Geometry: final body of the model. Coordinates: model frame, mm. A direction names the side the tool comes from. Coordinates: 2 decimals unless noted, no trailing zeros. Order: outer loops, then holes, each group sorted by start corner. A loop starts at its lowest first (then second) coordinate and runs counter-clockwise, first axis right, second up. Notation, with made-up numbers: (44.5, 59) - (94.5, 59) arc R27 cw to (94.5, 98) - close; hole circle Ø10 at (52, 87.5). An arc over 180 degrees is marked (long way). Use a Markdown table: item, result. Add a question column.
```python
from build123d import *
from build123d.topology import SkipClean

# Parameters (mm, degrees)
EXTRUDE_1_DEPTH        = 15
SKETCH_4_W             = 25
SKETCH_4_H             = 29
CUT_EXTRUDE_2_DEPTH    = 13
PATTERN_LINEAR_1_COUNT = 4
PATTERN_LINEAR_1_PITCH = 27
CUT_EXTRUDE_3_DEPTH    = 149.559752288
EXTRUDE_2_DEPTH        = 142
CUT_EXTRUDE_4_DEPTH    = 149.559752288
SKETCH_14_W            = 21
SKETCH_14_H            = 4
CUT_EXTRUDE_7_DEPTH    = 84.348665256
PATTERN_LINEAR_3_COUNT = 5
PATTERN_LINEAR_3_PITCH = 27
CUT_EXTRUDE_8_DEPTH    = 84.348665256
SKETCH_17_R            = 2.5
CUT_EXTRUDE_9_DEPTH    = 84.348665256
PATTERN_LINEAR_4_COUNT = 4
PATTERN_LINEAR_4_PITCH = 27
SKETCH_21_W            = 31
SKETCH_21_H            = 13
CUT_EXTRUDE_11_DEPTH   = 32
CUT_EXTRUDE_12_DEPTH   = 0.5
PATTERN_LINEAR_5_COUNT = 4
PATTERN_LINEAR_5_PITCH = 27
CUT_EXTRUDE_13_DEPTH   = 6


# Read off the part's stored shape, not the designer's step: 镜向1
with BuildPart() as part:
    # 草图3 → 凸台-拉伸1 (new body)
    with BuildSketch(Plane(origin=(0, 0, 0), x_dir=(1, 0, 0), z_dir=(0, 1, 0))):
        Polygon((0, 0), (-71, 0), (-71, 41), (71, 41), (71, 0), align=None)
    extrude(amount=EXTRUDE_1_DEPTH)

    # 草图4 → 切除-拉伸2 (cut)
    with BuildSketch(Plane(origin=(0, 0, 0), x_dir=(1, 0, 0), z_dir=(0, 1, 0))):
        with Locations((-56.5, 24.5)):
            Rectangle(SKETCH_4_W, SKETCH_4_H)
    cut_extrude_2 = extrude(amount=CUT_EXTRUDE_2_DEPTH, mode=Mode.SUBTRACT)

    # 阵列(线性)1: 切除-拉伸2 ×4
    with Locations(*[(i * PATTERN_LINEAR_1_PITCH, 0, 0) for i in range(1, PATTERN_LINEAR_1_COUNT)]):
        add(cut_extrude_2, mode=Mode.SUBTRACT)

    # 草图6 → 切除-拉伸3 (cut, through all)
    with BuildSketch(Plane(origin=(71, 0, 0), x_dir=(0, 0, -1), z_dir=(1, 0, 0))):
        Polygon((0, 15), (7.5, 15), (8, 15), (8, 2), (7.5, 2), (0, 2), align=None)
    extrude(amount=-CUT_EXTRUDE_3_DEPTH, mode=Mode.SUBTRACT)

    # 草图7 → 凸台-拉伸2 (add)
    with BuildSketch(Plane(origin=(71, 0, 0), x_dir=(0, 0, -1), z_dir=(1, 0, 0))):
        with BuildLine():
            Line((0, 0), (4, 0))
            ThreePointArc((4, 0), (2.828427125, -2.828427125), (0, -4))
            Line((0, -4), (0, 0))
        make_face()
    extrude(amount=-EXTRUDE_2_DEPTH)

    # 草图8 → 切除-拉伸4 (cut, through all)
    with BuildSketch(Plane(origin=(71, 0, 0), x_dir=(0, 0, -1), z_dir=(1, 0, 0))):
        with BuildLine():
            Line((0, -1), (0, -2))
            Line((0, -2), (0, -3))
            ThreePointArc((0, -3), (1, -2), (0, -1))
        make_face()
    extrude(amount=-CUT_EXTRUDE_4_DEPTH, mode=Mode.SUBTRACT)

    # 草图14 → 切除-拉伸7 (cut, through all)
    with BuildSketch(Plane.XY):
        with Locations((-56.5, -2)):
            Rectangle(SKETCH_14_W, SKETCH_14_H)
    cut_extrude_7 = extrude(amount=-CUT_EXTRUDE_7_DEPTH, mode=Mode.SUBTRACT)

    # 阵列(线性)3: 切除-拉伸7 ×5
    with Locations(*[(i * PATTERN_LINEAR_3_PITCH, 0, 0) for i in range(1, PATTERN_LINEAR_3_COUNT)]):
        add(cut_extrude_7, mode=Mode.SUBTRACT)

    # 草图16 → 切除-拉伸8 (cut, through all)
    with BuildSketch(Plane.XY):
        Polygon((71, -1), (71, 0), (42.178247133, 0), (42.178247133, -4), (71, -4), align=None)
    extrude(amount=-CUT_EXTRUDE_8_DEPTH, mode=Mode.SUBTRACT)

    # 草图17 → 切除-拉伸9 (cut, through all)
    with BuildSketch(Plane.XZ):
        with Locations(Location((-56.5, -4, 0), (0, 0, 270))):
            Circle(SKETCH_17_R)
    cut_extrude_9 = extrude(amount=-CUT_EXTRUDE_9_DEPTH, mode=Mode.SUBTRACT)

    # 阵列(线性)4: 切除-拉伸9 ×4
    with Locations(*[(i * PATTERN_LINEAR_4_PITCH, 0, 0) for i in range(1, PATTERN_LINEAR_4_COUNT)]):
        add(cut_extrude_9, mode=Mode.SUBTRACT)

    # 草图21 → 切除-拉伸11 (cut)
    with BuildSketch(Plane(origin=(71, 0, 0), x_dir=(0, 0, -1), z_dir=(1, 0, 0))):
        with Locations((23.5, 8.5)):
            Rectangle(SKETCH_21_W, SKETCH_21_H)
    extrude(amount=-CUT_EXTRUDE_11_DEPTH, mode=Mode.SUBTRACT)

    # 草图23 → 切除-拉伸12 (cut)
    with BuildSketch(Plane(origin=(0, 0, -41), x_dir=(-1, 0, 0), z_dir=(0, 0, -1))):
        Polygon((55.25, 2.9), (56.5, 2.9), (57.75, 2.9), (57.75, 3.5), (57.75, 4.1), (55.25, 4.1), (55.25, 3.5), align=None)
    cut_extrude_12 = extrude(amount=-CUT_EXTRUDE_12_DEPTH, mode=Mode.SUBTRACT)

    # 阵列(线性)5: 切除-拉伸12 ×4
    with Locations(*[(i * PATTERN_LINEAR_5_PITCH, 0, 0) for i in range(1, PATTERN_LINEAR_5_COUNT)]):
        add(cut_extrude_12, mode=Mode.SUBTRACT)

    # 镜向1: part across plane


with BuildPart() as part_1:
    with SkipClean():  # the faces are left unmerged after this step: merging them gives an invalid solid
        add(part.part)
        add(part.part.mirror(Plane.XY))

    # 草图25 → 切除-拉伸13 (cut)
    with SkipClean():  # the faces are left unmerged after this step: merging them gives an invalid solid
        with BuildSketch(Plane(origin=(71, 0, 0), x_dir=(0, 0, -1), z_dir=(1, 0, 0))):
            Polygon((41, 15), (41, 0), (-41, 0), (-41, 15), (-39, 15), (-39, 2), (39, 2), (39, 15), align=None)
        extrude(amount=-CUT_EXTRUDE_13_DEPTH, mode=Mode.SUBTRACT)


solid = part_1.part
```
1) Draft query along Z for faces 6 (the flat face through (35, -0.7, -0.1)), 7 (the flat face through (24, 6, 10)), 8 (the flat face through (-3, 6, -39)). Return one class per face: released by +Z, released by -Z, zero draft, split by the parting line, or undercut.
2) Section query A-A (y = 8.5). Give the number of separate pieces and of enclosed holes in the cut face, and give its area (3 significant figures).
3) Section query B-B (z = 21.5). Return the cut outline in (x, y), and give its area (3 significant figures).
4) Access query for faces 1 (the flat face through (39, 9, 23)), 2 (the cylindrical face through (-4.94, 0.99, -3.46)), 3 (the flat face through (-13, -0.7, -0.1)), 4 (the flat face through (-3, 13, -25)), 5 (the flat face through (-15, 9, -8)). Directions: +Z, -Z, +X, -X, +Y, -Y. A direction counts if a zero-diameter tool reaches every point of the face in a straight line with its end or side. Return the directions, or none.
5) Line query: line 1 (Z direction, x = 6, y = 7.75); line 2 (X direction, y = 5, z = -24.5); line 3 (X direction, y = 0.5, z = 4). Output: solid intervals per line, ascending. Write a range as from..to.
6) First-contact query: pin 1 (1.5 mm diameter, centred on y = 12.5, z = -13.5, fed in from +X); pin 2 (6 mm diameter, centred on x = 47.5, z = 6, fed in from +Y); pin 3 (3 mm diameter, centred on x = 11.5, z = -15, fed in from -Y). Flat tips, straight axial feed; report the tip coordinate or a pass-through.
From the geometry:
| question | item | result |
|---|---|---|
| 1 | face 6 | zero draft |
| 1 | face 7 | undercut |
| 1 | face 8 | undercut |
| 2 | separate pieces | 2 |
| 2 | enclosed holes | 8 |
| 2 | area | 1,560 mm^2 |
| 3 | outline | (-71, 0) - (-69, 0) - (-69, 13) - (-44, 13) - (-44, 0) - (-42, 0) - (-42, 13) - (-17, 13) - (-17, 0) - (-15, 0) - (-15, 13) - (10, 13) - (10, 0) - (12, 0) - (12, 13) - (37, 13) - (37, 0) - (65, 0) - (65, 2) - (39, 2) - (39, 15) - (-71, 15) - close |
| 3 | area | 402 mm^2 |
| 4 | face 1 | +X, +Y |
| 4 | face 2 | +Y, -Y |
| 4 | face 3 | +Z, -Z, -Y |
| 4 | face 4 | -Y |
| 4 | face 5 | +X, -X, +Y |
| 5 | line 1 | z = -41..-39, -10..-8, 8..10, 39..41 |
| 5 | line 2 | x = -71..-69, -44..-42, -17..-15, 10..12, 37..39 |
| 5 | line 3 | x = -71..-59, -54..-32, -27..-5, 0..22, 27..65 |
| 6 | pin 1 | stops at x = 39 |
| 6 | pin 2 | stops at y = 2 |
| 6 | pin 3 | stops at y = 0 |
